from build123d import *

# Parameters (mm, degrees)
SKETCH1_R                = 1.5875
BOSS_EXTRUDE1_DEPTH      = 6.35
BOSS_EXTRUDE1_DEPTH_BACK = 31.304
SKETCH2_R                = 1.5875
CUT_EXTRUDE1_DEPTH       = 7.654
SKETCH3_R                = 0.750000024
CUT_EXTRUDE2_DEPTH       = 12.7
CUT_EXTRUDE2_TAPER       = 1


with BuildPart() as part:
    # Sketch1 → Boss-Extrude1 (new body, two sides)
    with BuildSketch(Plane.XY) as boss_extrude1_sk:
        Circle(SKETCH1_R)
    extrude(amount=BOSS_EXTRUDE1_DEPTH)
    extrude(boss_extrude1_sk.sketch, amount=-BOSS_EXTRUDE1_DEPTH_BACK)

    # Sketch2 → Cut-Extrude1 (cut)
    with BuildSketch(Plane(origin=(0, 0, -31.304), x_dir=(-1, 0, 0), z_dir=(0, 0, -1))):
        Circle(SKETCH2_R)
    extrude(amount=-CUT_EXTRUDE1_DEPTH, mode=Mode.SUBTRACT)

    # Sketch3 → Cut-Extrude2 (cut)
    with BuildSketch(Plane.XY.offset(6.35)):
        Circle(SKETCH3_R)
    extrude(amount=-CUT_EXTRUDE2_DEPTH, taper=CUT_EXTRUDE2_TAPER, mode=Mode.SUBTRACT)


solid = part.part
Can you work these out from the model? Positions are in its coordinate system, mm. A direction names the side the tool comes from. Coordinates: 2 decimals unless noted, no trailing zeros. Loops run counter-clockwise (first coordinate to the right, second up) from the corner with the lowest first, then second, coordinate; pieces in that order, holes last. Notation, with made-up numbers: (-6, 28) - (31, 28) arc R11 cw to (31, 42) - close; hole circle Ø3 at (43.25, -4.75). An arc over 180 degrees is marked (long way). Put each result on its own line as item: value. Start each with the question number.
Item 1: If I drill on line 1 along Y through (x, z) = (0.1, -20); line 2 along X through (y, z) = (1.4, 2); line 3 along Y through (x, z) = (0.4, 3), over which ranges is the centre line in solid material (lowest first)?
Item 2: Which directions (+Z, -Z, +X, -X, +Y, -Y) give clear straight access to the entire face, cutting with the end or side of a thin tool? Please do faces 4 (the face through (-0.506, -0.388, -0.089)), 5 (the face through (1, 0, 6.35)).
Item 3: Suppose I cut it at C-C (x = 1.1). Please give me the cut outline in (y, z).
Item 4: Suppose I cut it at A-A (z = -1.5). Please give me the cut outline in (x, y) (1 decimal).
Item 5: Suppose I cut it at D-D (y = 1.25). Please give me the cut outline in (x, z).
Item 6: If we mould it in two halves opening along X, with no side actions, what happens to faces 1 (the face through (0, 0, -6.35)), 2 (the face through (0, 0, -23.65)), 3 (the face through (-0.34, -1.55, -8.44))? For each: +X half, -X half, draft (parallel to the pull), parting line (faces both ways), or undercut.
Item 7: For pin 1 (1.5 mm diameter, centred on x = -0.5, y = 0, fed in from +Z), with a flat end and sliding along its axis, tell me the tip position at first contact or that it passes through.
Item 8: Suppose I cut it at B-B (z = -10). Please give me the cut outline in (x, y) (1 decimal), and give its area (3 significant figures).
Here are the results:
1. line 1: -1.58 to 1.58
1. line 2: -0.75 to 0.75
1. line 3: -1.54 to -0.56, 0.56 to 1.54
2. face 4: +Z
2. face 5: +Z, +X, -X, +Y, -Y
3. outline: (-1.14, -23.65) - (1.14, -23.65) - (1.14, 6.35) - (-1.14, 6.35) - close
4. outline: circle Ø3.2 at (0, 0); hole circle Ø1.2 at (0, 0)
5. outline: (-0.98, -23.65) - (0.98, -23.65) - (0.98, 6.35) - (-0.98, 6.35) - close
6. face 1: undercut
6. face 2: draft
6. face 3: parting line
7. pin 1: z = 6.35
8. outline: circle Ø3.2 at (0, 0)
8. area: 7.92 mm²
